The model under review builds one solid part; all positions refer to its coordinate system, in mm. A direction names the side the tool comes from. Round coordinates to 2 decimals unless told otherwise and drop trailing zeros. Write each loop counter-clockwise with the first axis right and the second up, starting at its lowest first coordinate (ties: lowest second). Pieces come first, ordered by that corner, then holes. Notation, with made-up numbers: (70, -36.75) -> (99, -36.75) arc R17 cw to (99, -20.75) -> close; hole circle Ø6 at (-8, -10.5). An arc over 180 degrees is marked (long way). Answer as a JSON object with one key per item and string values. Group by question number.
1) We need section A-A, the plane z = 8. Write out the cut boundary in (x, y), then the cut area to 3 significant figures.
2) To check wall thickness, follow probe 1 along X at (y, z) = (10.5, -45); probe 2 along X at (y, z) = (1.5, 42.5); probe 3 along Z at (x, y) = (-53, 21.25). State the ranges of each line that lie inside material, in increasing order. Write a range as [from, to].
3) Mouldability with a two-part tool opening along X and no side actions: class faces 1 (the flat face through (63.5, 13, -27)), 2 (the flat face through (1, 2.54, 24)), 3 (the flat face through (1, 13, 50.8)) as pulls with the +X half, pulls with the -X half, needs draft (parallel to the pull), parting line crosses it, or undercut.
4) Insertion check: pin 1 Ø8 at (x, z) = (12, -121) entering from -Y; pin 2 Ø24 at (x, z) = (10.5, 32.5) entering from +Y; pin 3 Ø5 at (x, z) = (44, -88.5) entering from -Y. Each pin has a flat end and moves straight along its axis. Give the tip position at first contact, or say it passes through.
5) Machinability: for faces 4 (the flat face through (-60.96, 16, -27)), 5 (the flat face through (61.4, 25.4, -96.4)), which of the approach directions +Z, -Z, +X, -X, +Y, -Y give a long, thin tool a straight path to every point of the face, cutting with its end or side? Answer none if there is none.
from build123d import *

# Parameters (mm, degrees)
BOSS_EXTRUDE1_DEPTH = 63.5
SHELL1_T            = -2.54
SKETCH4_W           = 12.7
SKETCH4_H           = 44.45
CUT_EXTRUDE1_DEPTH  = 168.042419907


with BuildPart() as part:
    # Sketch1 → Boss-Extrude1 (new, symmetric)
    with BuildSketch(Plane(origin=(0, 0, 0), x_dir=(0, 0, -1), z_dir=(1, 0, 0))):
        with BuildLine():
            Line((-50.8, 25.4), (-50.8, 0))
            Line((-50.8, 0), (0, 0))
            add(Edge.make_bspline(
                [(0, 0), (90.399909762, 0.128526821), (138.872298675, 8.862290589), (152.4, 25.4)],
                knots=[0, 0, 0, 0, 1, 1, 1, 1], degree=3))
            Line((152.4, 25.4), (-50.8, 25.4))
        make_face()
    extrude(amount=BOSS_EXTRUDE1_DEPTH, both=True)

    # Shell1
    shell1_openings = [part.faces().sort_by_distance(p)[0] for p in [
        (0, 25.4, -50.8),
    ]]
    offset(amount=SHELL1_T, openings=shell1_openings, kind=Kind.INTERSECTION)

    # Sketch4 → Cut-Extrude1 (cut, through all)
    with BuildSketch(Plane(origin=(0, 25.4, 0), x_dir=(1, 0, 0), z_dir=(0, 1, 0))):
        with Locations((-54.61, -26.035)):
            Rectangle(SKETCH4_W, SKETCH4_H)
        with Locations((54.61, -26.035)):
            Rectangle(SKETCH4_W, SKETCH4_H)
    extrude(amount=-CUT_EXTRUDE1_DEPTH, mode=Mode.SUBTRACT)


solid = part.part
Here are the results:
{
 "1": {"outline": "(-63.5, 0) -> (-60.96, 0) -> (-60.96, 25.4) -> (-63.5, 25.4) -> close; (-48.26, 0) -> (48.26, 0) -> (48.26, 2.54) -> (-48.26, 2.54) -> close; (60.96, 0) -> (63.5, 0) -> (63.5, 25.4) -> (60.96, 25.4) -> close", "area": "374 mm^2"},
 "2": {"probe 1": "x = [-63.5, -60.96], [60.96, 63.5]", "probe 2": "x = [-63.5, -60.96], [-48.26, 48.26], [60.96, 63.5]", "probe 3": "z = [-148.06, -143.59], [48.26, 50.8]"},
 "3": {"face 1": "pulls with the +X half", "face 2": "undercut", "face 3": "needs draft"},
 "4": {"pin 1": "stops at y = 8.9", "pin 2": "stops at y = 2.54", "pin 3": "stops at y = 3.91"},
 "5": {"face 4": "+Y", "face 5": "+Z, -Z, +X, -X, +Y"}
}
